Part model, mm, in its own coordinate system. Face numbers are marked on the shaded views. A direction names the side the tool comes from. Coordinates: 2 decimals unless noted, no trailing zeros. Write each loop counter-clockwise with the first axis right and the second up, starting at its lowest first coordinate (ties: lowest second). Pieces come first, ordered by that corner, then holes. Notation, with made-up numbers: (-32.75, 41) -> (11.25, 41) arc R33 ccw to (11.25, 72) -> close; hole circle Ø8 at (12.25, 0). An arc over 180 degrees is marked (long way). Write item = value, one per line. Start each with the question number.
Q1. Band-saw the part on B-B, the plane x = 149. List the corners of the cut face in (y, z).
Q2. Pin check, flat tips, straight feed: P1, Ø8.5, axis at y = -24, z = 0.5, coming from the -X side; P2, Ø8, axis at y = -29.5, z = -14.5, coming from the +X side; P3, Ø4, axis at y = -24, z = -20.5, coming from the -X side; P4, Ø2, axis at y = -0.5, z = -22, coming from the -X side. Stop position of each tip, or through.
Q3. Pull direction Z, two halves, no side cores. Call the marked faces 1 and 2: released by +Z, released by -Z, zero draft, split by the parting line, or undercut.
Q4. Tool access for the marked faces 3, 4, 5 and 6: list every direction of +Z, -Z, +X, -X, +Y, -Y with a clear straight run to the whole face (end or side of a thin tool).
Q5. Band-saw the part on A-A, the plane x = -8. List the corners of the cut face in (y, z), plus the area to 3 significant figures.
Q6. Probe line 1 (X direction, y = -12, z = -0.5); line 2 (X direction, y = -25, z = -20); line 3 (X direction, y = 3.5, z = -12.5). List the from-to ranges inside material, lowest first.
from build123d import *

# Parameters (mm, degrees)
CUT_EXTRUDE1_START = -5
SKETCH2_R          = 27
SKETCH2_R_2        = 8.4
CUT_EXTRUDE1_DEPTH = 5
SKETCH3_R          = 27
SKETCH3_R_2        = 8.4
CUT_EXTRUDE2_DEPTH = 5
SKETCH4_R          = 1.5
CUT_EXTRUDE3_DEPTH = 5
CUT_EXTRUDE4_START = -5
SKETCH6_R          = 1.5
CUT_EXTRUDE4_DEPTH = 5


with BuildPart() as part:
    # Sketch1 → Revolve1 (revolve)
    with BuildSketch(Plane.XY, mode=Mode.PRIVATE) as revolve1_sk:
        Polygon((136.652683421, -10.294425689), (136.652683421, -14.294425689), (145.975223156, -14.294425689), (145.975223156, -15.694425689), (175.475223156, -15.694425689), (175.475223156, -22.694425689), (-64.527316579, -22.694425689), (-64.527316579, -15.694425689), (-35.027316579, -15.694425689), (-35.027316579, -14.294425689), (-25.707316579, -14.294425689), (-25.707316579, -10.294425689), (-14.707316579, -10.294425689), (-14.707316579, -14.294425689), (15.472683421, -14.294425689), (15.472683421, 8.449285256), (20.472683421, 8.449285256), (20.472683421, 9.949285256), (90.472683421, 9.949285256), (90.475230364, 8.449287418), (95.475223156, 8.457777227), (95.475223156, -14.294425689), (125.652683421, -14.294425689), (125.652683421, -10.294425689), align=None)
    revolve(revolve1_sk.sketch.rotate(Axis((-64.527316579, -22.694425689, 0), (1, 0, 0)), 180), axis=Axis((-64.527316579, -22.694425689, 0), (1, 0, 0)))

    # Sketch2 → Cut-Extrude1 (cut)
    with BuildSketch(Plane.ZY.offset(-15.472683421).offset(CUT_EXTRUDE1_START)):
        with Locations(Location((0, -22.694425689, 0), (0, 0, 270))):
            Circle(SKETCH2_R)
        with Locations(Location((0, -22.694425689, 0), (0, 0, 270))):
            Circle(SKETCH2_R_2, mode=Mode.SUBTRACT)
    extrude(amount=CUT_EXTRUDE1_DEPTH, mode=Mode.SUBTRACT)

    # Sketch3 → Cut-Extrude2 (cut)
    with BuildSketch(Plane(origin=(95.475223156, 0, 0), x_dir=(0, 0, -1), z_dir=(1, 0, 0))):
        with Locations(Location((0, -22.694425689, 0), (0, 0, 270))):
            Circle(SKETCH3_R)
        with Locations(Location((0, -22.694425689, 0), (0, 0, 270))):
            Circle(SKETCH3_R_2, mode=Mode.SUBTRACT)
    extrude(amount=-CUT_EXTRUDE2_DEPTH, mode=Mode.SUBTRACT)

    # Sketch4 → Cut-Extrude3 (cut)
    with BuildSketch(Plane.ZY.offset(64.527316579)):
        with Locations(Location((0, -22.694425689, 0), (0, 0, 270))):
            Circle(SKETCH4_R)
    extrude(amount=-CUT_EXTRUDE3_DEPTH, mode=Mode.SUBTRACT)

    # Sketch6 → Cut-Extrude4 (cut)
    with BuildSketch(Plane(origin=(175.475223156, 0, 0), x_dir=(0, 0, -1), z_dir=(1, 0, 0)).offset(CUT_EXTRUDE4_START)):
        with Locations(Location((0, -22.694425689, 0), (0, 0, 270))):
            Circle(SKETCH6_R)
    extrude(amount=CUT_EXTRUDE4_DEPTH, mode=Mode.SUBTRACT)


solid = part.part
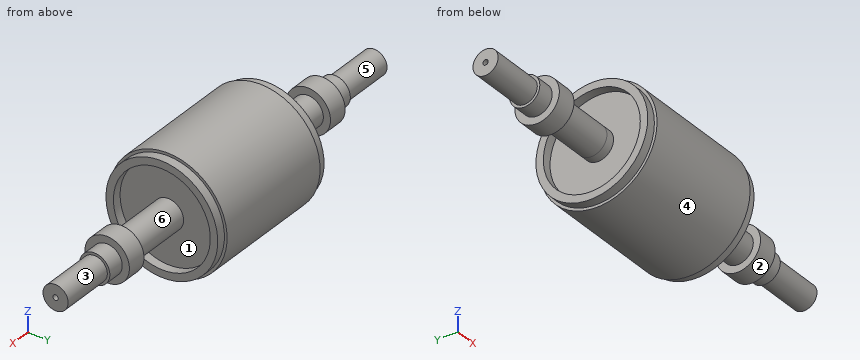
Ans:
q1.outline = circle Ø14 at (-22.69, 0)
q2.P1 = -64.53
q2.P2 = 136.65
q2.P3 = 20.47
q2.P4 = 15.47
q3.face_1 = undercut
q3.face_2 = split by the parting line
q4.face_3 = +X
q4.face_4 = +X, -X
q4.face_5 = -X
q4.face_6 = none
q5.outline = circle Ø16.8 at (-22.69, 0)
q5.area = 222 mm2
q6.line_1 = -25.71 to -14.71, 20.47 to 90.48, 125.65 to 136.65
q6.line_2 = 20.47 to 90.48
q6.line_3 = 15.47 to 95.48
